Source: CAD feature listing. Evaluate the final solid. Frame: model axes, mm. Face numbers are marked on the shaded views. A direction names the side the tool comes from. Round coordinates to 2 decimals unless told otherwise and drop trailing zeros. Loops run counter-clockwise (first coordinate to the right, second up) from the corner with the lowest first, then second, coordinate; pieces in that order, holes last. Notation, with made-up numbers: (-20, 1) - (9, 1) arc R8 cw to (9, 16) - close; hole circle Ø9 at (69, 84.25). An arc over 180 degrees is marked (long way). One line per question, with ' | ' between items. Start each with the question number.
1. Access query for the marked faces 1 and 2. Directions: +Z, -Z, +X, -X, +Y, -Y. A direction counts if a zero-diameter tool reaches every point of the face in a straight line with its end or side. Return the directions, or none.
2. Pin query (flat end, axial travel): pin 1 (8 mm diameter, centred on x = -106.5, y = 59, fed in from +Z); pin 2 (6 mm diameter, centred on x = -89, y = 75, fed in from -Z); pin 3 (3 mm diameter, centred on y = 76, z = 31, fed in from +X). Return the tip coordinate at first contact, or that it passes through.
3. Cut plane B-B (z = 37). Return loops of the section in (x, y).
4. Cut plane A-A (x = -54.5). Return loops of the section in (y, z).
5. Ray query, line 1 (Z direction, x = -59, y = 52.5); line 2 (Z direction, x = -58.5, y = 18); line 3 (Z direction, x = -84, y = 41). Return the intervals inside material, ascending.
6. Cut plane C-C (x = -14). Return loops of the section in (y, z), then the cut area to 3 significant figures.
7. Mould query, pull axis X, two halves, no side actions, for the marked faces 3, 4 and 5. Classes: pulls with the +X half, pulls with the -X half, needs draft (parallel to the pull), parting line crosses it, or undercut.
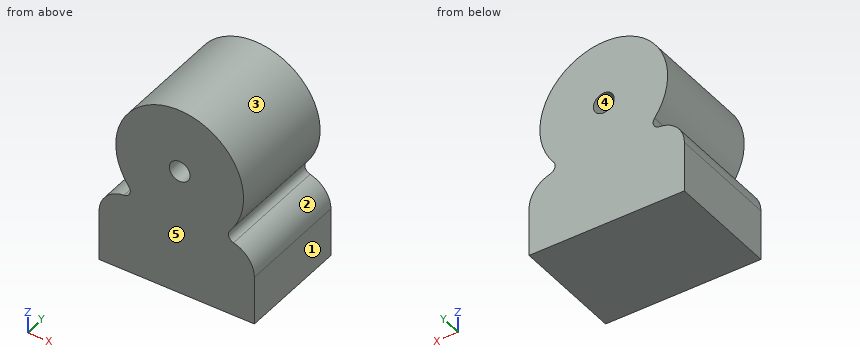
```python
from build123d import *

# Parameters (mm, degrees)
F1_DEPTH = 101.6
F3_D     = 19.05
F4_R     = 25.4
F5_R     = 6.35


with BuildPart() as f1:
    # F0 (on Front) → F1 (new body)
    with BuildSketch(Plane.XZ):
        with BuildLine():
            Line((-130.225047, 48.010781), (-130.225047, -24.027621))
            Line((-130.225047, -24.027621), (12.208596, -22.256413))
            Line((12.208596, -22.256413), (12.208596, 48.010781))
            Line((12.208596, 48.010781), (-19.5011, 48.010781))
            ThreePointArc((-19.5011, 48.010781), (-56.295205, 152.231707), (-93.08931, 48.010781))
            Line((-93.08931, 48.010781), (-130.225047, 48.010781))
        make_face()
    extrude(amount=-F1_DEPTH)

    # F3 (through all)
    with Locations(Plane.XZ):
        with Locations((-56.295205, 93.626358)):
            Hole(F3_D / 2)

    # F4
    f4_edges = [f1.edges().sort_by_distance(p)[0] for p in [
        (-130.225047, 50.8, 48.010781),
        (12.208596, 50.8, 48.010781),
    ]]
    fillet(f4_edges, radius=F4_R)

    # F5
    f5_edges = [f1.edges().sort_by_distance(p)[0] for p in [
        (-19.5011, 50.8, 48.010781),
        (-93.08931, 50.8, 48.010781),
    ]]
    fillet(f5_edges, radius=F5_R)


solid = f1.part
```
Answers follow:
1) face 1: +Z, -Z, +X, +Y, -Y | face 2: +X, +Y, -Y
2) pin 1: stops at z = 129.68 | pin 2: stops at z = -23.55 | pin 3: stops at x = 11.26
3) outline: (-125.76, 0) - (7.74, 0) - (7.74, 101.6) - (-125.76, 101.6) - close
4) outline: (0, -23.09) - (101.6, -23.09) - (101.6, 84.27) - (0, 84.27) - close; (0, 102.98) - (101.6, 102.98) - (101.6, 152.2) - (0, 152.2) - close
5) line 1: z = -23.14 to 84.49, 102.76 to 152.17 | line 2: z = -23.14 to 84.36, 102.89 to 152.19 | line 3: z = -23.45 to 145.27
6) outline: (0, -22.58) - (101.6, -22.58) - (101.6, 134.19) - (0, 134.19) - close | area: 15,900 mm2
7) face 3: parting line crosses it | face 4: undercut | face 5: needs draft
